Read the model definition and answer for the solid it produces. Units are mm, in the model's axes. A direction names the side the tool comes from. Round coordinates to 2 decimals unless told otherwise and drop trailing zeros. Order: outer loops, then holes, each group sorted by start corner. A loop starts at its lowest first (then second) coordinate and runs counter-clockwise, first axis right, second up. Notation, with made-up numbers: (-10.75, 19.5) - (3.25, 19.5) arc R7 cw to (3.25, 30.5) - close; hole circle Ø9 at (11.25, 60). An arc over 180 degrees is marked (long way). Put each result on its own line as item: value. Start each with the question number.
Q1. Each of these flat-tipped pins is pushed along its axis until it touches: pin 1 Ø2 at (x, z) = (-5.5, 4.5) entering from -Y; pin 2 Ø0.6 at (y, z) = (2.5, 4.5) entering from -X; pin 3 Ø1.6 at (x, z) = (3, 4) entering from +Y. Where does it stop, or does it pass through?
Q2. Section A-A on z = 3.7 is taken. Give the vertices of the cut face in (x, y).
Q3. Find the intervals of material crossed by line 1 along Y through (x, z) = (-6.5, 3.25); line 2 along Y through (x, z) = (1.5, 2.1); line 3 along X through (y, z) = (1, 2.1), in increasing order. Write a range as from..to.
Q4. Section C-C on y = -1 is taken. Give the vertices of the cut face in (x, z).
Q5. Section B-B on x = -2.5 is taken. Give the vertices of the cut face in (y, z).
Q6. Section D-D on y = -5.5 is taken. Give the vertices of the cut face in (x, z), then the cut area to 4 significant figures.
Q7. Which of the six approach directions +Z, -Z, +X, -X, +Y, -Y give full straight-line access (tool end or side, diameter ignored) to faces 1 (the face through (0, 0, 2)), 2 (the face through (-20.25, 3, 4)), 3 (the face through (20.25, -3, 4))?
Q8. For a pull along X with two mould halves and no side action, classify faces 4 (the face through (0, -7, 1)), 5 (the face through (20.25, 0, 2.5)), 6 (the face through (-25.25, 0, 1)), 7 (the face through (20.25, 3, 4)) as pulls with the +X half, pulls with the -X half, needs draft (parallel to the pull), parting line crosses it, or undercut.
from build123d import *

# Parameters (mm, degrees)
F0_W     = 40.5
F0_H     = 4.1
F1_DEPTH = 2
F0_H_2   = 1.95
F2_DEPTH = 5
F0_W_2   = 50.5
F0_H_3   = 14
F3_DEPTH = 3


with BuildPart() as f1:
    # F0 (on Top) → F1 (new body)
    with BuildSketch(Plane.XY):
        Rectangle(F0_W, F0_H)
    extrude(amount=F1_DEPTH)

    # F0 (on Top) → F2 (join)
    with BuildSketch(Plane.XY):
        with Locations((0, 3.025)):
            Rectangle(F0_W, F0_H_2)
        with Locations((0, -3.025)):
            Rectangle(F0_W, F0_H_2)
    extrude(amount=F2_DEPTH)

    # F0 (on Top) → F3 (join)
    with BuildSketch(Plane.XY):
        Rectangle(F0_W_2, F0_H_3)
        Polygon((-20.25, 2.05), (-20.25, 4), (20.25, 4), (20.25, 2.05), (20.25, -2.05), (20.25, -4), (-20.25, -4), (-20.25, -2.05), align=None, mode=Mode.SUBTRACT)
    extrude(amount=F3_DEPTH)


solid = f1.part
Findings:
1. pin 1: y = -4
1. pin 2: x = -20.25
1. pin 3: y = 4
2. outline: (-20.25, -4) - (20.25, -4) - (20.25, -2.05) - (-20.25, -2.05) - close; (-20.25, 2.05) - (20.25, 2.05) - (20.25, 4) - (-20.25, 4) - close
3. line 1: -4..-2.05, 2.05..4
3. line 2: -7..-2.05, 2.05..7
3. line 3: -25.25..-20.25, 20.25..25.25
4. outline: (-25.25, 0) - (25.25, 0) - (25.25, 3) - (20.25, 3) - (20.25, 2) - (-20.25, 2) - (-20.25, 3) - (-25.25, 3) - close
5. outline: (-7, 0) - (7, 0) - (7, 3) - (4, 3) - (4, 5) - (2.05, 5) - (2.05, 2) - (-2.05, 2) - (-2.05, 5) - (-4, 5) - (-4, 3) - (-7, 3) - close
6. outline: (-25.25, 0) - (25.25, 0) - (25.25, 3) - (-25.25, 3) - close
6. area: 151.5 mm2
7. face 1: +Z
7. face 2: +Z, -X, +Y, -Y
7. face 3: +Z, +X, +Y, -Y
8. face 4: needs draft
8. face 5: undercut
8. face 6: pulls with the -X half
8. face 7: pulls with the +X half
